```python
from build123d import *

# Parameters (mm, degrees)
SKETCH1_W           = 75
SKETCH1_H           = 21
BOSS_EXTRUDE1_DEPTH = 4
SKETCH2_W           = 8
SKETCH2_H           = 4
BOSS_EXTRUDE2_DEPTH = 6
SKETCH3_W           = 10
SKETCH3_H           = 4
BOSS_EXTRUDE3_DEPTH = 4
LPATTERN1_COUNT     = 4
LPATTERN1_PITCH     = 20
SKETCH4_W           = 1
SKETCH4_H           = 4
BOSS_EXTRUDE4_DEPTH = 4
SKETCH5_W           = 45
SKETCH5_H           = 4
SKETCH5_W_2         = 10
BOSS_EXTRUDE5_DEPTH = 4
SKETCH6_R           = 1.75
CUT_EXTRUDE1_DEPTH  = 85.864598037


with BuildPart() as part:
    # Sketch1 → Boss-Extrude1 (new body)
    with BuildSketch(Plane(origin=(0, 0, 0), x_dir=(1, 0, 0), z_dir=(0, 1, 0))):
        with Locations((37.5, -10.5)):
            Rectangle(SKETCH1_W, SKETCH1_H)
    extrude(amount=BOSS_EXTRUDE1_DEPTH)

    # Sketch2 → Boss-Extrude2 (add)
    with BuildSketch(Plane(origin=(75, 0, 0), x_dir=(0, 0, -1), z_dir=(1, 0, 0))):
        with Locations((-17, 2)):
            Rectangle(SKETCH2_W, SKETCH2_H)
        with Locations((-4, 2)):
            Rectangle(SKETCH2_W, SKETCH2_H)
    extrude(amount=BOSS_EXTRUDE2_DEPTH)

    # Sketch3 → Boss-Extrude3 (add, through all)
    with BuildSketch(Plane(origin=(0, 4, 0), x_dir=(1, 0, 0), z_dir=(0, 1, 0))):
        with Locations((66, 2)):
            Rectangle(SKETCH3_W, SKETCH3_H)
    boss_extrude3 = extrude(amount=-BOSS_EXTRUDE3_DEPTH)

    # LPattern1: Boss-Extrude3 ×4
    with Locations(*[(-i * LPATTERN1_PITCH, 0, 0) for i in range(1, LPATTERN1_COUNT)]):
        add(boss_extrude3)

    # Sketch4 → Boss-Extrude4 (add, through all)
    with BuildSketch(Plane(origin=(0, 4, 0), x_dir=(1, 0, 0), z_dir=(0, 1, 0))):
        with Locations((0.5, 2)):
            Rectangle(SKETCH4_W, SKETCH4_H)
    extrude(amount=-BOSS_EXTRUDE4_DEPTH)

    # Sketch5 → Boss-Extrude5 (add, through all)
    with BuildSketch(Plane(origin=(0, 4, 0), x_dir=(1, 0, 0), z_dir=(0, 1, 0))):
        with Locations((22.5, -23)):
            Rectangle(SKETCH5_W, SKETCH5_H)
        with Locations((60, -23)):
            Rectangle(SKETCH5_W_2, SKETCH5_H)
    extrude(amount=-BOSS_EXTRUDE5_DEPTH)

    # Sketch6 → Cut-Extrude1 (cut, through all)
    with BuildSketch(Plane(origin=(0, 4, 0), x_dir=(1, 0, 0), z_dir=(0, 1, 0))):
        with Locations(Location((12, -13, 0), (0, 0, 270))):
            Circle(SKETCH6_R)
    extrude(amount=-CUT_EXTRUDE1_DEPTH, mode=Mode.SUBTRACT)


solid = part.part
```
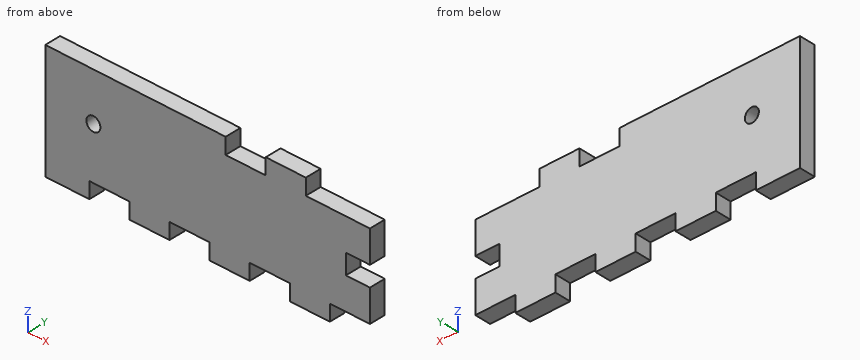
Part model, mm, in its own coordinate system. Round coordinates to 2 decimals unless told otherwise and drop trailing zeros. Loops run counter-clockwise (first coordinate to the right, second up) from the corner with the lowest first, then second, coordinate; pieces in that order, holes last.
Item 1: Cut at C-C, the plane z = 9.75. Give the cut face in (x, y), then the cut area to 3 significant figures.
Item 2: Drop flat-ended pins along their axis: P1, Ø2, axis at x = 79, y = 2, coming from the -Z side; P2, Ø3, axis at x = 12, z = 13, coming from the +Y side; P3, Ø1.2, axis at x = 69.5, y = 2, coming from the +Z side. Give the stop position or say it passes through.
Item 3: Cut at B-B, the plane x = 12. Give the cut face in (y, z), then the cut area to 3 significant figures.
Item 4: Drill centre lines: line 1 (X direction, y = 0.6, z = 9.5); line 2 (X direction, y = 1.6, z = 12.5); line 3 (Z direction, x = 58, y = 1.8). Where is each one in solid material? Low to high.
A:
1. outline: (0, 0) - (75, 0) - (75, 4) - (0, 4) - close
1. area: 300 mm2
2. P1: stops at z = 0
2. P2: passes through
2. P3: stops at z = 21
3. outline: (0, 0) - (4, 0) - (4, 11.25) - (0, 11.25) - close; (0, 14.75) - (4, 14.75) - (4, 25) - (0, 25) - close
3. area: 86.0 mm2
4. line 1: x = 0 to 75
4. line 2: x = 0 to 10.32, 13.68 to 75
4. line 3: z = 0 to 25
